from build123d import *

# Parameters (mm, degrees)
BOSS_EXTRUDE1_DEPTH = 30
SHELL2_T            = 8
SKETCH2_W           = 15
SKETCH2_H           = 23
CUT_EXTRUDE1_DEPTH  = 8
SKETCH3_W           = 15
SKETCH3_H           = 3
CUT_EXTRUDE2_DEPTH  = 5
SKETCH4_W           = 39.3748274
SKETCH4_H           = 39.3748274
SKETCH4_R           = 15
BOSS_EXTRUDE2_DEPTH = 40
CUT_EXTRUDE3_START  = -3
CUT_EXTRUDE3_DEPTH  = 3
CIRPATTERN1_COUNT   = 4


with BuildPart() as part:
    # Sketch1 → Boss-Extrude1 (new body)
    with BuildSketch(Plane(origin=(0, 0, 0), x_dir=(1, 0, 0), z_dir=(0, 1, 0))):
        Polygon((-50, 0), (50, 0), (50, 30), (7.5, 150), (-7.5, 150), (-50, 30), align=None)
    extrude(amount=BOSS_EXTRUDE1_DEPTH)

    # Shell2
    shell2_openings = [part.faces().sort_by_distance(p)[0] for p in [
        (0, 30, -56.96969697),
    ]]
    offset(amount=SHELL2_T, openings=shell2_openings, kind=Kind.INTERSECTION)

    # Sketch2 → Cut-Extrude1 (cut)
    with BuildSketch(Plane(origin=(0, -8, 0), x_dir=(-1, 0, 0), z_dir=(0, -1, 0))):
        with Locations((0, 138.5)):
            Rectangle(SKETCH2_W, SKETCH2_H)
    extrude(amount=-CUT_EXTRUDE1_DEPTH, mode=Mode.SUBTRACT)

    # Sketch3 → Cut-Extrude2 (cut)
    with BuildSketch(Plane.XY.offset(-150)):
        with Locations((0, 1.5)):
            Rectangle(SKETCH3_W, SKETCH3_H)
    extrude(amount=-CUT_EXTRUDE2_DEPTH, mode=Mode.SUBTRACT)

    # Sketch4 → Boss-Extrude2 (add)
    with BuildSketch(Plane.ZY.offset(58)):
        with Locations((-11.6874137, -27.6874137)):
            Rectangle(SKETCH4_W, SKETCH4_H)
        with Locations((-11.6874137, -27.6874137)):
            Circle(SKETCH4_R, mode=Mode.SUBTRACT)
    extrude(amount=-BOSS_EXTRUDE2_DEPTH)

    # Sketch5 → Cut-Extrude3 (cut)
    with BuildSketch(Plane(origin=(-18, 0, 0), x_dir=(0, 0, -1), z_dir=(1, 0, 0)).offset(CUT_EXTRUDE3_START)):
        with BuildLine():
            Line((27.950869668, -15.66659842), (24.201038889, -19.416429198))
            ThreePointArc((24.201038889, -19.416429198), (22.294015418, -17.080811982), (19.958398202, -15.173788511))
            Line((19.958398202, -15.173788511), (23.70822898, -11.423957733))
            ThreePointArc((23.70822898, -11.423957733), (27.950869668, -11.423957733), (27.950869668, -15.66659842))
        make_face()
    cut_extrude3 = extrude(amount=CUT_EXTRUDE3_DEPTH, mode=Mode.SUBTRACT)

    # CirPattern1: Cut-Extrude3 ×4 about axis
    cirpattern1_axis = Axis((0, -27.6874137, -11.6874137), (1, 0, 0))
    for i in range(1, CIRPATTERN1_COUNT):
        add(cut_extrude3.rotate(cirpattern1_axis, i * 360 / CIRPATTERN1_COUNT), mode=Mode.SUBTRACT)


solid = part.part
Work out the finished part from the listing and answer in its coordinate system (mm). A direction names the side the tool comes from. Give positions to 0.01 mm unless a question says otherwise; leave off trailing zeros. Loops run counter-clockwise (first coordinate to the right, second up) from the corner with the lowest first, then second, coordinate; pieces in that order, holes last. Notation, with made-up numbers: (24.25, 35.25) - (47.25, 35.25) arc R37 ccw to (47.25, 72.25) - close; hole circle Ø7 at (45, -38). An arc over 180 degrees is marked (long way). Answer in a Markdown table with one row per item.
(1) Consider L1, parallel to Y at x = 10.5, z = -117.5; L2, parallel to X at y = 14.5, z = -86.5; L3, parallel to X at y = 2.5, z = -83.5. Determine where each line is inside the solid, lowest interval first. Write a range as [from, to].
Results list:
| item | result |
|---|---|
| L1 | y = [-8, 0] |
| L2 | x = [-38.48, -29.99], [29.99, 38.48] |
| L3 | x = [-39.54, -31.05], [31.05, 39.54] |
(2) Section A-A (y = 11) is taken. Give the vertices of the cut face in (x, z).
Results list:
| item | result |
|---|---|
| outline | (-58, -31.37) - (-13.15, -158) - (13.15, -158) - (58, -31.37) - (58, 8) - (-58, 8) - close; hole (-50, -30) - (-7.5, -150) - (7.5, -150) - (50, -30) - (50, 0) - (-50, 0) - close |
(3) Section C-C (y = -31) is taken. Give the vertices of the cut face in (x, z).
Results list:
| item | result |
|---|---|
| outline | (-58, -31.37) - (-18, -31.37) - (-18, -26.32) - (-58, -26.32) - close; (-58, 2.94) - (-18, 2.94) - (-18, 8) - (-58, 8) - close |
(4) For a pull along Z with two mould halves and no side action, classify faces 4 (the face through (-21, -15, 1)), 5 (the face through (-35, 30, -75)) as pulls with the +Z half, pulls with the -Z half, needs draft (parallel to the pull), parting line crosses it, or undercut.
Results list:
| item | result |
|---|---|
| face 4 | undercut |
| face 5 | needs draft |
(5) A tool of negligible diameter and unlimited length cuts with its end or side. For faces 1 (the face through (-19.52, -37.81, -26.05)), 2 (the face through (-50, 15, -15)), 3 (the face through (0, 0, -152)), from which of +Z, -Z, +X, -X, +Y, -Y can it reach the whole face along a straight path? Write none if from no direction.
Results list:
| item | result |
|---|---|
| face 1 | +X |
| face 2 | +Y |
| face 3 | none |
(6) Section B-B (x = -28) is taken. Give the vertices of the cut face in (y, z), and give its area (3 significant figures).
Results list:
| item | result |
|---|---|
| outline | (-47.37, -31.37) - (-8, -31.37) - (-8, -116.08) - (30, -116.08) - (30, -92.12) - (0, -92.12) - (0, 0) - (30, 0) - (30, 8) - (-47.37, 8) - close; hole circle Ø30 at (-27.69, -11.69) |
| area | 2,800 mm² |
(7) Flat-ended cylindrical pins translate along their axes: pin 1 Ø4 at (x, z) = (22, -14) entering from -Y; pin 2 Ø1 at (x, z) = (17.5, -100.5) entering from +Y; pin 3 Ø6.5 at (y, z) = (-5.5, -142.5) entering from -X. Find the tip coordinate at first contact, or state that the pin passes through.
Results list:
| item | result |
|---|---|
| pin 1 | stops at y = -8 |
| pin 2 | stops at y = 0 |
| pin 3 | stops at x = -19.79 |
(8) Section D-D (z = -132.5) is taken. Give the vertices of the cut face in (x, y).
Results list:
| item | result |
|---|---|
| outline | (-22.18, -8) - (-7.5, -8) - (-7.5, 0) - (-13.7, 0) - (-13.7, 30) - (-22.18, 30) - close; (7.5, -8) - (22.18, -8) - (22.18, 30) - (13.7, 30) - (13.7, 0) - (7.5, 0) - close |
